Part model, mm, in its own coordinate system. Give positions to 0.01 mm unless a question says otherwise; leave off trailing zeros. Write each loop counter-clockwise with the first axis right and the second up, starting at its lowest first coordinate (ties: lowest second). Pieces come first, ordered by that corner, then holes. Notation, with made-up numbers: (-0.75, -1.5) - (48.25, -1.5) arc R23 cw to (48.25, 8.5) - close; hole circle Ø6 at (-34.5, 69). An arc over 180 degrees is marked (long way). Answer as a JSON object with one key per item and string values. Group by question number.
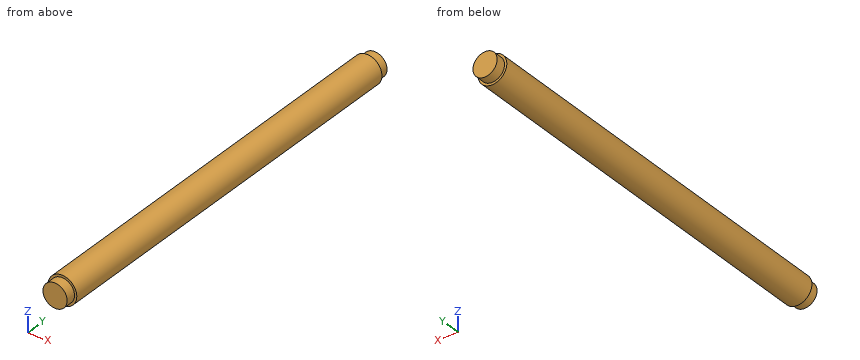
```python
from build123d import *

# Parameters (mm, degrees)
F0_R     = 14.859199
F1_DEPTH = 433.5
F2_R     = 14.859199
F2_R_2   = 12.5
F3_DEPTH = 10
F4_R     = 14.859199
F4_R_2   = 12.5
F5_DEPTH = 10


with BuildPart() as f1:
    # F0 (on Front) → F1 (new body)
    with BuildSketch(Plane.XZ):
        Circle(F0_R)
    extrude(amount=F1_DEPTH)

    # F2 (on face) → F3 (cut)
    with BuildSketch(Plane(origin=(0, 0, 0), x_dir=(-1, 0, 0), z_dir=(0, 1, 0))):
        Circle(F2_R)
        Circle(F2_R_2, mode=Mode.SUBTRACT)
    extrude(amount=-F3_DEPTH, mode=Mode.SUBTRACT)

    # F4 (on face) → F5 (cut)
    with BuildSketch(Plane.XZ.offset(433.5)):
        Circle(F4_R)
        Circle(F4_R_2, mode=Mode.SUBTRACT)
    extrude(amount=-F5_DEPTH, mode=Mode.SUBTRACT)


solid = f1.part
```
1) Drill centre lines: line 1 along Y through (x, z) = (12.75, 4); line 2 along Z through (x, y) = (-1, -136.5); line 3 along Z through (x, y) = (0, -80.5). Where is each one in solid material? Low to high. Write a range as from..to.
2) Saw through at A-A (x = -2.5). List the corners of the cut face in (y, z).
3) Saw through at B-B (z = -6.25). List the corners of the cut face in (x, y).
4) Saw through at C-C (y = -162). List the corners of the cut face in (x, z), and give its area (3 significant figures).
5) Drop flat-ended pins along their axis: P1, Ø1.5, axis at x = -7, y = -101, coming from the -Z side; P2, Ø2, axis at x = -6.5, y = -364.5, coming from the +Z side; P3, Ø1.5, axis at x = -11, y = -233.5, coming from the +Z side. Give the stop position or say it passes through.
Checks:
{
 "1": {"line 1": "-423.5..-10", "line 2": "-14.83..14.83", "line 3": "-14.86..14.86"},
 "2": {"outline": "(-433.5, -12.25) - (-423.5, -12.25) - (-423.5, -14.65) - (-10, -14.65) - (-10, -12.25) - (0, -12.25) - (0, 12.25) - (-10, 12.25) - (-10, 14.65) - (-423.5, 14.65) - (-423.5, 12.25) - (-433.5, 12.25) - close"},
 "3": {"outline": "(-13.48, -423.5) - (-10.83, -423.5) - (-10.83, -433.5) - (10.83, -433.5) - (10.83, -423.5) - (13.48, -423.5) - (13.48, -10) - (10.83, -10) - (10.83, 0) - (-10.83, 0) - (-10.83, -10) - (-13.48, -10) - close"},
 "4": {"outline": "circle Ø29.72 at (0, 0)", "area": "694 mm2"},
 "5": {"P1": "z = -13.48", "P2": "z = 13.8", "P3": "z = 10.76"}
}
